For this review, take the finished solid that the model builds, in its own axes (mm). A direction names the side the tool comes from. Coordinates: 2 decimals unless noted, no trailing zeros. Order: outer loops, then holes, each group sorted by start corner. A loop starts at its lowest first (then second) coordinate and runs counter-clockwise, first axis right, second up.
from build123d import *

# Parameters (mm, degrees)
BOSS_EXTRUDE1_DEPTH             = 71.58
CUT_EXTRUDE2_DEPTH              = 136.85530183
CUT_EXTRUDE2_DEPTH_BACK         = 136.85530183
CUT_EXTRUDE3_DEPTH              = 136.85530183
CUT_EXTRUDE3_DEPTH_BACK         = 136.85530183
CUT_EXTRUDE4_DEPTH              = 136.85530183
CUT_EXTRUDE4_DEPTH_BACK         = 136.85530183
SKETCH16_R                      = 5
CUT_EXTRUDE11_DEPTH             = 136.85530183
SKETCH17_W                      = 45
SKETCH17_H                      = 69.61
BOSS_EXTRUDE2_DEPTH             = 6
SKETCH18_R                      = 4.9
BOSS_EXTRUDE3_DEPTH             = 10
CUT_EXTRUDE12_REACH             = 151.101
CUT_EXTRUDE12_DIRECTION_2_REACH = 151.101
BOSS_EXTRUDE4_REACH             = 150.692


with BuildPart() as part:
    # Sketch2 → Boss-Extrude1 (new body)
    with BuildSketch(Plane(origin=(0, 0, 0), x_dir=(0, 0, -1), z_dir=(1, 0, 0))):
        Polygon((-35.251160643, -109.956001694), (34.358839357, -109.956001694), (33.316287702, -102.063950804), (29.698839357, 5.004872941), (24.583736048, 63.004872941), (-20.256263952, 63.004872941), (-35.251160643, 5.004872941), (-27.753712298, -102.063950804), align=None)
    extrude(amount=BOSS_EXTRUDE1_DEPTH)

    # Sketch4 → Cut-Extrude2 (cut, two sides: drawn at the far end of the back side and taken through both)
    with BuildSketch(Plane.XY.offset(-CUT_EXTRUDE2_DEPTH_BACK)):
        Polygon((58.29, -109.956001694), (71.58, 5.004872941), (71.58, -109.956001694), align=None)
        Polygon((0, 5.004872941), (13.29, -109.956001694), (0, -109.956001694), align=None)
    extrude(amount=CUT_EXTRUDE2_DEPTH + CUT_EXTRUDE2_DEPTH_BACK, mode=Mode.SUBTRACT)

    # Sketch5 → Cut-Extrude3 (cut, two sides: drawn at the far end of the back side and taken through both)
    with BuildSketch(Plane.XY.offset(-CUT_EXTRUDE3_DEPTH_BACK)):
        Polygon((0, 5.004872941), (0, 63.004872941), (0.75, 63.004872941), align=None)
        Polygon((71.58, 63.004872941), (70.83, 63.004872941), (71.58, 5.004872941), align=None)
    extrude(amount=CUT_EXTRUDE3_DEPTH + CUT_EXTRUDE3_DEPTH_BACK, mode=Mode.SUBTRACT)

    # Sketch9 → Cut-Extrude4 (cut, two sides: drawn at the far end of the back side and taken through both)
    with BuildSketch(Plane.XY.offset(-CUT_EXTRUDE4_DEPTH_BACK)):
        Polygon((3.25, 63.004872941), (68.33, 63.004872941), (68.705, 5.004872941), (2.875, 5.004872941), align=None)
    extrude(amount=CUT_EXTRUDE4_DEPTH + CUT_EXTRUDE4_DEPTH_BACK, mode=Mode.SUBTRACT)

    # Sketch16 → Cut-Extrude11 (cut, through all)
    with BuildSketch(Plane(origin=(0, 0, 0), x_dir=(0, 0, -1), z_dir=(1, 0, 0))):
        with Locations(Location((1.149194348, 48.404872941, 0), (0, 0, 90))):
            Circle(SKETCH16_R)
    extrude(amount=CUT_EXTRUDE11_DEPTH, mode=Mode.SUBTRACT)

    # Sketch17 → Boss-Extrude2 (add)
    with BuildSketch(Plane.XZ.offset(109.956001694)):
        with Locations((35.79, 0.446160643)):
            Rectangle(SKETCH17_W, SKETCH17_H)
    extrude(amount=BOSS_EXTRUDE2_DEPTH)

    # Sketch18 → Boss-Extrude3 (add)
    with BuildSketch(Plane.XZ.offset(115.956001694)):
        with Locations(Location((35.79, 0.446160643, 0), (0, 0, 270))):
            Circle(SKETCH18_R)
    extrude(amount=BOSS_EXTRUDE3_DEPTH)

    # Cut-Extrude12: up to this plane
    cut_extrude12_end = Plane(origin=(71.58, -102.063950804, -33.316287702), z_dir=(0, -0.03376692966076465, 0.999429734629346))
    # Sketch19 → Cut-Extrude12 (cut, up to the surface)
    with BuildSketch(Plane.XY, mode=Mode.PRIVATE) as cut_extrude12_sk1:
        Polygon((2.875, 5.004872941), (7.892261572, -41.495127059), (63.687738428, -41.495127059), (68.705, 5.004872941), align=None)
    cut_extrude12_tool1 = split(extrude(cut_extrude12_sk1.sketch, amount=-CUT_EXTRUDE12_REACH, mode=Mode.PRIVATE), bisect_by=cut_extrude12_end, keep=Keep.BOTH, mode=Mode.PRIVATE)
    add(cut_extrude12_tool1.solids().sort_by_distance((35.79, -17.605725, 0))[0], mode=Mode.SUBTRACT)

    # Cut-Extrude12 direction 2: up to this plane
    cut_extrude12_direction_2_end = Plane(origin=(71.58, 5.004872941, 35.251160643), z_dir=(0, 0.06985351817200207, -0.9975572595089436))
    # Sketch19 → Cut-Extrude12 direction 2 (cut, up to the surface)
    with BuildSketch(Plane.XY, mode=Mode.PRIVATE) as cut_extrude12_direction_2_sk1:
        Polygon((2.875, 5.004872941), (7.892261572, -41.495127059), (63.687738428, -41.495127059), (68.705, 5.004872941), align=None)
    cut_extrude12_direction_2_tool1 = split(extrude(cut_extrude12_direction_2_sk1.sketch, amount=CUT_EXTRUDE12_DIRECTION_2_REACH, mode=Mode.PRIVATE), bisect_by=cut_extrude12_direction_2_end, keep=Keep.BOTH, mode=Mode.PRIVATE)
    add(cut_extrude12_direction_2_tool1.solids().sort_by_distance((35.79, -17.605725, 0))[0], mode=Mode.SUBTRACT)

    # Boss-Extrude4: up to this plane
    boss_extrude4_end = Plane(origin=(63.687738428, -41.495127059, -111.104129622), z_dir=(0.9942293381213047, -0.10727545487609211, 0))
    # Sketch20 → Boss-Extrude4 (add, up to the surface)
    with BuildSketch(Plane(origin=(3.375716186, 0.364233357, 0), x_dir=(0, 0, -1), z_dir=(0.9942293381213048, 0.10727545487609252, 0)), mode=Mode.PRIVATE) as boss_extrude4_sk1:
        Polygon((29.698839357, 4.667574579), (-31.995018137, -42.102318661), (31.269897506, -42.102318661), align=None)
    boss_extrude4_tool1 = split(extrude(boss_extrude4_sk1.sketch, amount=BOSS_EXTRUDE4_REACH, dir=(1, 0, 0), mode=Mode.PRIVATE), bisect_by=boss_extrude4_end, keep=Keep.BOTH, mode=Mode.PRIVATE)
    add(boss_extrude4_tool1.solids().sort_by_distance((6.219841, -25.995127, -9.657906))[0])


solid = part.part
1. The part is to be moulded in two halves that separate along X. For faces 1 (the face through (37.782, -17.727, 0.461)), 2 (the face through (64.84, -53.28, -0.04)), 3 (the face through (1.6, 34.41, 27.65)), say which applies: +X half, -X half, draft (parallel to the pull), parting line (faces both ways), or undercut.
Answer below:
face 1: undercut
face 2: +X half
face 3: draft
2. Machinability: for faces 4 (the face through (35.462, -106.065, -33.845)), 5 (the face through (35.462, -105.955, 31.45)), which of the approach directions +Z, -Z, +X, -X, +Y, -Y give a long, thin tool a straight path to every point of the face, cutting with its end or side? Answer none if there is none.
Answer below:
face 4: -Z, +X, -X, +Y
face 5: +Z, +X, -X
3. Take a section at B-B, the plane x = 18. Give the boundary of the cut face in (y, z), plus the area to 3 significant figures.
Answer below:
outline: (-115.96, -34.36) - (-109.96, -34.36) - (-102.06, -33.32) - (5, -29.7) - (-41.5, 32) - (-102.06, 27.75) - (-109.96, 35.25) - (-115.96, 35.25) - close
area: 6,170 mm2
4. Take a section at A-A, the plane z = 30. Give the boundary of the cut face in (x, y) (3 decimals).
Answer below:
outline: (0, 5.005) - (8.669, -69.985) - (62.911, -69.985) - (71.58, 5.005) - (71.317, 25.316) - (68.574, 25.316) - (68.705, 5.005) - (63.85, -39.991) - (7.73, -39.991) - (2.875, 5.005) - (3.006, 25.316) - (0.263, 25.316) - close; (12.651, -104.428) - (13.29, -109.956) - (13.29, -115.956) - (58.29, -115.956) - (58.29, -109.956) - (58.929, -104.428) - close
5. Clearance check with flat-ended pins moving along their axes: pin 1 Ø3 at (y, z) = (-112.5, 4.5) entering from +X; pin 2 Ø6 at (y, z) = (12.5, -19) entering from -X; pin 3 Ø2 at (y, z) = (3.5, -9) entering from +X. State where each tip first meets the part, or that it passes through.
Answer below:
pin 1: stops at x = 58.29
pin 2: stops at x = 0.06
pin 3: stops at x = 71.52
6. To check wall thickness, follow L1, parallel to X at y = -102, z = -25.5; L2, parallel to X at y = 24, z = -15.5; L3, parallel to X at y = 13.5, z = -27. State the ranges of each line that lie inside material, in increasing order.
Answer below:
L1: x = 12.37 to 59.21
L2: x = 0.25 to 3, 68.58 to 71.33
L3: x = 0.11 to 2.93, 68.65 to 71.47
7. Take a section at D-D, the plane z = 14. Give the boundary of the cut face in (x, y) (3 decimals).
Answer below:
outline: (0, 5.005) - (13.29, -109.956) - (13.29, -115.956) - (58.29, -115.956) - (58.29, -109.956) - (71.58, 5.005) - (70.83, 63.005) - (68.33, 63.005) - (68.705, 5.005) - (65.151, -27.932) - (6.429, -27.932) - (2.875, 5.005) - (3.25, 63.005) - (0.75, 63.005) - close
8. Take a section at C-C, the plane y = -38.5. Give the boundary of the cut face in (x, z), plus the area to 3 significant figures.
Answer below:
outline: (5.03, -31.17) - (66.55, -31.17) - (66.55, 32.2) - (64.01, 32.2) - (64.01, 28.02) - (7.57, 28.02) - (7.57, 32.2) - (5.03, 32.2) - close
area: 3,660 mm2
